Geometry: final body of the model. Coordinates: model frame, mm. Face numbers are marked on the shaded views. A direction names the side the tool comes from. Coordinates: 2 decimals unless noted, no trailing zeros. Loops run counter-clockwise (first coordinate to the right, second up) from the corner with the lowest first, then second, coordinate; pieces in that order, holes last. Notation, with made-up numbers: (58.25, 57.25) -> (96.25, 57.25) arc R22 cw to (96.25, 78.25) -> close; hole circle Ø5 at (33.5, -15). An arc over 180 degrees is marked (long way). One line per item, written item: value. Start each with the question number.
Item 1: Set-up query: the marked faces 1 and 2. Return all of +Z, -Z, +X, -X, +Y, -Y with unobstructed straight access to the full face (end or side cutting, diameter ignored); none if empty.
Item 2: Section query A-A on x = 0. Return loops of the section in (y, z), then the cut area to 3 significant figures.
Item 3: Section query B-B on y = -24.13. Return loops of the section in (x, z), then the cut area to 3 significant figures.
Item 4: Ray query, probe 1 along Y at (x, z) = (17, 12.25); probe 2 along X at (y, z) = (0, 5.5); probe 3 along X at (y, z) = (18.5, 2.5). Return the intervals inside material, ascending. Write a range as from..to.
Item 5: Section query D-D on z = 11.25. Give the number of separate pieces and of enclosed holes in the cut face, then the cut area to 3 significant figures.
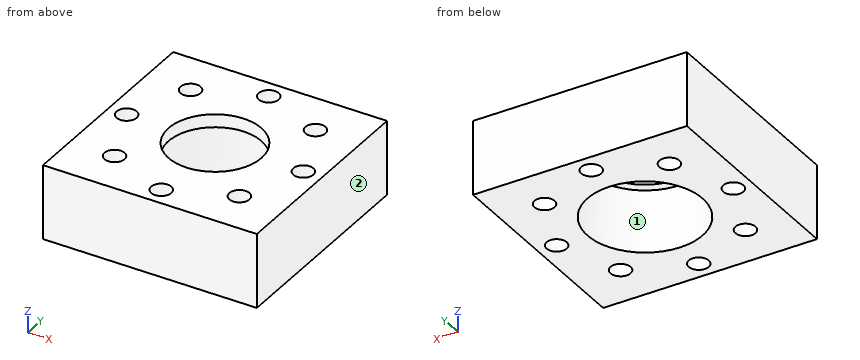
from build123d import *

# Parameters (mm, degrees)
SKETCH1_W                = 58.42
SKETCH1_H                = 58.42
BOSS_EXTRUDE1_DEPTH      = 20.32
M5_CLEARANCE_HOLE1_D     = 5.5
M5_CLEARANCE_HOLE1_DEPTH = 20.32
CIRPATTERN1_COUNT        = 8
SKETCH9_R                = 14.4907
SKETCH9_R_2              = 12.7
BOSS_EXTRUDE2_DEPTH      = 3.556


with BuildPart() as part:
    # Sketch1 → Boss-Extrude1 (new body)
    with BuildSketch(Plane.XY):
        Rectangle(SKETCH1_W, SKETCH1_H)
    extrude(amount=BOSS_EXTRUDE1_DEPTH)

    # Sketch7 → 1 NPT Tapped Hole2 (revolve, cut)
    with BuildSketch(Plane.YZ):
        Polygon((0, 0), (0, 20.32), (14.4907, 20.32), (14.4907, 16.764), (15.22797859, 16.764), (15.7299152, 0), align=None)
    revolve(axis=Axis((0, 0, -6.35), (0, 0, 1)), mode=Mode.SUBTRACT)

    # M5 Clearance Hole1
    with Locations(Plane(origin=(0, 0, 0), x_dir=(-1, 0, 0), z_dir=(0, 0, -1))):
        with Locations((0, 24.13)):
            m5_clearance_hole1 = Hole(M5_CLEARANCE_HOLE1_D / 2, depth=M5_CLEARANCE_HOLE1_DEPTH)

    # CirPattern1: M5 Clearance Hole1 ×8 about axis
    cirpattern1_axis = Axis((0, 0, 0), (0, 0, 1))
    for i in range(1, CIRPATTERN1_COUNT):
        add(m5_clearance_hole1.rotate(cirpattern1_axis, i * 360 / CIRPATTERN1_COUNT), mode=Mode.SUBTRACT)

    # Sketch9 → Boss-Extrude2 (add)
    with BuildSketch(Plane.XY.offset(20.32)):
        Circle(SKETCH9_R)
        Circle(SKETCH9_R_2, mode=Mode.SUBTRACT)
    extrude(amount=-BOSS_EXTRUDE2_DEPTH)


solid = part.part
Reply:
1. face 1: -Z
1. face 2: +Z, -Z, +X, +Y, -Y
2. outline: (-29.21, 0) -> (-26.88, 0) -> (-26.88, 20.32) -> (-29.21, 20.32) -> close; (-21.38, 0) -> (-15.73, 0) -> (-15.23, 16.76) -> (-12.7, 16.76) -> (-12.7, 20.32) -> (-21.38, 20.32) -> close; (12.7, 16.76) -> (15.23, 16.76) -> (15.73, 0) -> (21.38, 0) -> (21.38, 20.32) -> (12.7, 20.32) -> close; (26.88, 0) -> (29.21, 0) -> (29.21, 20.32) -> (26.88, 20.32) -> close
2. area: 354 mm²
3. outline: (-29.21, 0) -> (-2.75, 0) -> (-2.75, 20.32) -> (-29.21, 20.32) -> close; (2.75, 0) -> (29.21, 0) -> (29.21, 20.32) -> (2.75, 20.32) -> close
3. area: 1,080 mm²
4. probe 1: y = -29.21..-19.81, -14.31..14.31, 19.81..29.21
4. probe 2: x = -29.21..-26.88, -21.38..-15.57, 15.57..21.38, 26.88..29.21
4. probe 3: x = -29.21..-19.41, -14.72..14.72, 19.41..29.21
5. separate pieces: 1
5. enclosed holes: 9
5. area: 2,480 mm²
